Check sheet for the modelled part. Datum: model origin and axes. Units: mm. Face numbers are marked on the shaded views. A direction names the side the tool comes from. Give positions to 0.01 mm unless a question says otherwise; leave off trailing zeros. Order: outer loops, then holes, each group sorted by start corner. A loop starts at its lowest first (then second) coordinate and runs counter-clockwise, first axis right, second up. Notation, with made-up numbers: M 88,-18.5 L 102,-18.5 A28 ccw 102,17.5 Z; hole C 63,45 d11. An arc over 180 degrees is marked long. Answer in a Markdown table with one row per item. Add a question column.
from build123d import *

# Parameters (mm, degrees)
SKETCH1_R           = 12.7
BOSS_EXTRUDE1_DEPTH = 5.08
SKETCH2_R           = 0.762
CUT_EXTRUDE1_DEPTH  = 19.66511184
SKETCH3_R           = 4.7625
BOSS_EXTRUDE2_DEPTH = 4.7625
SKETCH4_R           = 2.5146
CUT_EXTRUDE2_DEPTH  = 21.480595847
SKETCH5_R           = 0.79375
CUT_EXTRUDE3_DEPTH  = 24.964415416


with BuildPart() as part:
    # Sketch1 → Boss-Extrude1 (new body)
    with BuildSketch(Plane.XY):
        Circle(SKETCH1_R)
    extrude(amount=BOSS_EXTRUDE1_DEPTH)

    # Sketch2 → Cut-Extrude1 (cut, through all)
    with BuildSketch(Plane.XY.offset(5.08)):
        with Locations((-8.45058, 0)):
            Circle(SKETCH2_R)
        with Locations((8.45058, 0)):
            Circle(SKETCH2_R)
    extrude(amount=-CUT_EXTRUDE1_DEPTH, mode=Mode.SUBTRACT)

    # Sketch3 → Boss-Extrude2 (add)
    with BuildSketch(Plane.XY.offset(5.08)):
        with Locations(Location((0, 0, 0), (0, 0, 180))):
            Circle(SKETCH3_R)
    extrude(amount=BOSS_EXTRUDE2_DEPTH)

    # Sketch4 → Cut-Extrude2 (cut, through all)
    with BuildSketch(Plane.XY.offset(9.8425)):
        Circle(SKETCH4_R)
    extrude(amount=-CUT_EXTRUDE2_DEPTH, mode=Mode.SUBTRACT)

    # Sketch5 → Cut-Extrude3 (cut, through all)
    with BuildSketch(Plane(origin=(0, 5.08, 0), x_dir=(1, 0, 0), z_dir=(0, 1, 0))):
        with Locations(Location((0, -7.413542721, 0), (0, 0, 270))):
            Circle(SKETCH5_R)
    extrude(amount=-CUT_EXTRUDE3_DEPTH, mode=Mode.SUBTRACT)


solid = part.part
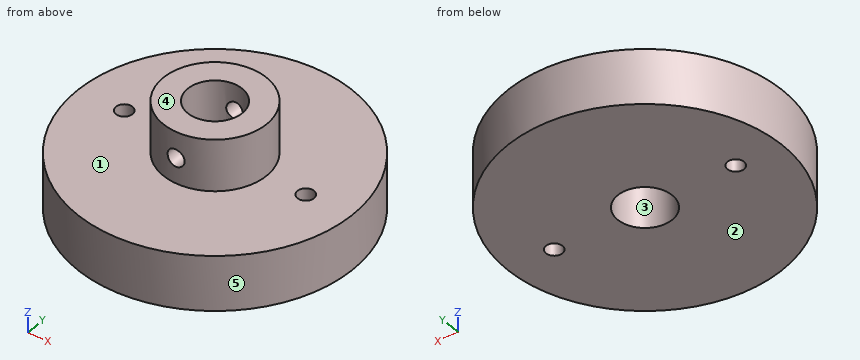
Q1. Cross-section at D-D (z = 3.25). Record the boundary of the cut face in (x, y), and give its area (3 significant figures).
Q2. Thickness scan on probe 1 along Z at (x, y) = (0, -3.3); probe 2 along Z at (x, y) = (4.75, 4.25); probe 3 along Y at (x, z) = (0.5, 4.75). Record the ranges inside material, lowest first.
Q3. Cross-section at A-A (y = 0). Record the boundary of the cut face in (x, z), and give its area (3 significant figures).
Q4. Go/stop test with flat-tipped pins: pin 1 (1 mm diameter, centred on y = -3, z = 2.5, fed in from +X); pin 2 (5 mm diameter, centred on x = 4, z = 5, fed in from -Y); pin 3 (1.2 mm diameter, centred on x = -8.45, y = 0, fed in from -Z); pin 4 (1.8 mm diameter, centred on x = 0, z = 7.41, fed in from +Y). Record where each tip stops, or that it passes through.
Q5. Cross-section at B-B (x = 0). Record the boundary of the cut face in (y, z).
Q6. Draft check along Y on the marked faces 3, 4 and 5. Enter one of: pulls with the +Y half, pulls with the -Y half, needs draft (parallel to the pull), parting line crosses it, or undercut.
Q7. Tool access check on the marked faces 1 and 2. Record the directions out of +Z, -Z, +X, -X, +Y, -Y that give a thin tool (end or side, any length) a straight path to the whole face; none if there is none.
Q8. Cross-section at C-C (z = 9). Record the boundary of the cut face in (x, y) (1 decimal), and give its area (3 significant figures).
Values follow:
| question | item | result |
|---|---|---|
| 1 | outline | C 0,0 d25.4; hole C -8.45,0 d1.52; hole C 0,0 d5.03; hole C 8.45,0 d1.52 |
| 1 | area | 483 mm² |
| 2 | probe 1 | 0 to 6.62, 8.21 to 9.84 |
| 2 | probe 2 | 0 to 5.08 |
| 2 | probe 3 | -12.69 to -2.46, 2.46 to 12.69 |
| 3 | outline | M -12.7,0 L -9.21,0 L -9.21,5.08 L -12.7,5.08 Z; M -7.69,0 L -2.51,0 L -2.51,9.84 L -4.76,9.84 L -4.76,5.08 L -7.69,5.08 Z; M 2.51,0 L 7.69,0 L 7.69,5.08 L 4.76,5.08 L 4.76,9.84 L 2.51,9.84 Z; M 9.21,0 L 12.7,0 L 12.7,5.08 L 9.21,5.08 Z |
| 3 | area | 109 mm² |
| 4 | pin 1 | x = 12.45 |
| 4 | pin 2 | y = -12.61 |
| 4 | pin 3 | through |
| 4 | pin 4 | y = 4.76 |
| 5 | outline | M -12.7,0 L -2.51,0 L -2.51,6.62 L -4.76,6.62 L -4.76,5.08 L -12.7,5.08 Z; M -4.76,8.21 L -2.51,8.21 L -2.51,9.84 L -4.76,9.84 Z; M 2.51,0 L 12.7,0 L 12.7,5.08 L 4.76,5.08 L 4.76,6.62 L 2.51,6.62 Z; M 2.51,8.21 L 4.76,8.21 L 4.76,9.84 L 2.51,9.84 Z |
| 6 | face 3 | undercut |
| 6 | face 4 | needs draft |
| 6 | face 5 | parting line crosses it |
| 7 | face 1 | +Z |
| 7 | face 2 | -Z, +X, -X, +Y, -Y |
| 8 | outline | C 0,0 d9.5; hole C 0,0 d5 |
| 8 | area | 51.4 mm² |
